Geometry: final body of the model. Coordinates: model frame, mm. Round coordinates to 2 decimals unless told otherwise and drop trailing zeros. Loops run counter-clockwise (first coordinate to the right, second up) from the corner with the lowest first, then second, coordinate; pieces in that order, holes last. Notation, with made-up numbers: (48.25, -28.5) -> (92.25, -28.5) arc R18 cw to (92.25, 1.5) -> close; hole circle Ø2 at (-38, -2.75). An arc over 180 degrees is marked (long way). Answer in a Markdown table with one row per item.
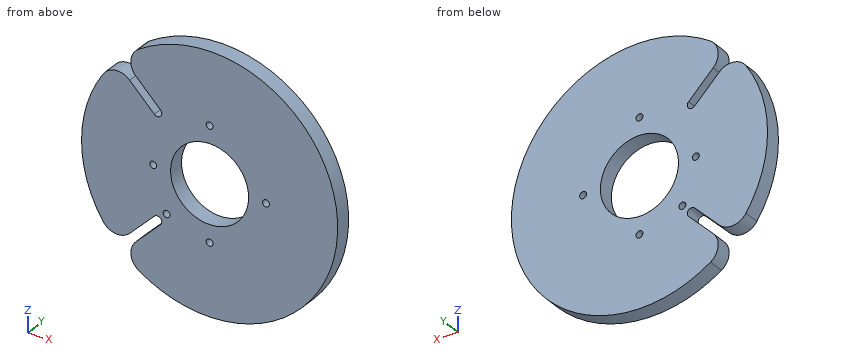
```python
from build123d import *

# Parameters (mm, degrees)
SKETCH1_R           = 75
BOSS_EXTRUDE1_DEPTH = 9.525
CUT_EXTRUDE2_REACH  = 108.493
FILLET1_R           = 10.16
SKETCH39_R          = 22.86
SKETCH39_R_2        = 2.0193
CUT_EXTRUDE30_DEPTH = 247.31360274
SKETCH42_R          = 2.0193
CUT_EXTRUDE33_DEPTH = 247.31360274


with BuildPart() as part:
    # Sketch1 → Boss-Extrude1 (new body)
    with BuildSketch(Plane(origin=(0, 0, 0), x_dir=(1, 0, 0), z_dir=(0, 1, 0))):
        with Locations(Location((0, 0, 0), (0, 0, 90))):
            Circle(SKETCH1_R)
    extrude(amount=BOSS_EXTRUDE1_DEPTH)

    # Sketch11 → Cut-Extrude2 (cut, up to next)
    with BuildSketch(Plane(origin=(0, 9.525, 0), x_dir=(1, 0, 0), z_dir=(0, 1, 0)), mode=Mode.PRIVATE) as cut_extrude2_sk1:
        with BuildLine():
            Line((-54.798637954, 51.206535505), (-32.347997651, 28.755895202))
            ThreePointArc((-32.347997651, 28.755895202), (-28.755895202, 28.755895202), (-28.755895202, 32.347997651))
            Line((-28.755895202, 32.347997651), (-51.206535505, 54.798637954))
            ThreePointArc((-51.206535505, 54.798637954), (-53.033008589, 53.033008589), (-54.798637954, 51.206535505))
        make_face()
    cut_extrude2_tool1 = extrude(cut_extrude2_sk1.sketch, amount=-CUT_EXTRUDE2_REACH, mode=Mode.PRIVATE) & part.part
    # Sketch11 → Cut-Extrude2 (cut, up to next)
    with BuildSketch(Plane(origin=(0, 9.525, 0), x_dir=(1, 0, 0), z_dir=(0, 1, 0)), mode=Mode.PRIVATE) as cut_extrude2_sk2:
        with BuildLine():
            Line((-51.206535505, -54.798637954), (-28.755895202, -32.347997651))
            ThreePointArc((-28.755895202, -32.347997651), (-28.755895202, -28.755895202), (-32.347997651, -28.755895202))
            Line((-32.347997651, -28.755895202), (-54.798637954, -51.206535505))
            ThreePointArc((-54.798637954, -51.206535505), (-53.033008589, -53.033008589), (-51.206535505, -54.798637954))
        make_face()
    cut_extrude2_tool2 = extrude(cut_extrude2_sk2.sketch, amount=-CUT_EXTRUDE2_REACH, mode=Mode.PRIVATE) & part.part
    add(cut_extrude2_tool1.solids().sort_by_distance((-41.078737, 9.525, -41.078737))[0], mode=Mode.SUBTRACT)
    add(cut_extrude2_tool2.solids().sort_by_distance((-41.078737, 9.525, 41.078737))[0], mode=Mode.SUBTRACT)

    # Fillet1
    fillet1_edges = [part.edges().sort_by_distance(p)[0] for p in [
        (-51.206535505, 4.7625, 54.798637954),
        (-54.798637954, 4.7625, 51.206535505),
        (-54.798637954, 4.7625, -51.206535505),
        (-51.206535505, 4.7625, -54.798637954),
    ]]
    fillet(fillet1_edges, radius=FILLET1_R)

    # Sketch39 → Cut-Extrude30 (cut, through all)
    with BuildSketch(Plane(origin=(-73.768816189, 9.525, -121.080352405), x_dir=(1, 0, 0), z_dir=(0, 1, 0))):
        with Locations(Location((73.768816189, -121.080352405, 0), (0, 0, 270))):
            Circle(SKETCH39_R)
        with Locations(Location((73.768816189, -88.060352405, 0), (0, 0, 270))):
            Circle(SKETCH39_R_2)
        with Locations(Location((106.788816189, -121.080352405, 0), (0, 0, 270))):
            Circle(SKETCH39_R_2)
        with Locations(Location((73.768816189, -154.100352405, 0), (0, 0, 270))):
            Circle(SKETCH39_R_2)
        with Locations(Location((40.748816189, -121.080352405, 0), (0, 0, 270))):
            Circle(SKETCH39_R_2)
    extrude(amount=-CUT_EXTRUDE30_DEPTH, mode=Mode.SUBTRACT)

    # Sketch42 → Cut-Extrude33 (cut, through all)
    with BuildSketch(Plane(origin=(-73.768816189, 9.525, -121.080352405), x_dir=(1, 0, 0), z_dir=(0, 1, 0))):
        with Locations(Location((48.605023435, -95.916559651, 0), (0, 0, 270))):
            Circle(SKETCH42_R)
    extrude(amount=-CUT_EXTRUDE33_DEPTH, mode=Mode.SUBTRACT)


solid = part.part
```
Item 1: Pin query (flat end, axial travel): pin 1 Ø1.5 at (x, y) = (-12, 7.5) entering from -Z; pin 2 Ø3 at (y, z) = (6, 43.5) entering from +X; pin 3 Ø5 at (y, z) = (1, 41.5) entering from -X; pin 4 Ø3 at (x, z) = (0, -33.02) entering from +Y. Return the tip coordinate at first contact, or that it passes through.
Answer:
| item | result |
|---|---|
| pin 1 | stops at z = -74.15 |
| pin 2 | stops at x = 62.14 |
| pin 3 | stops at x = -64.06 |
| pin 4 | passes through |
Item 2: Cut plane B-B (z = -21). Output: boundary loops of the cut face in (x, y) (3 decimals).
Answer:
| item | result |
|---|---|
| outline | (-72, 0) -> (-9.032, 0) -> (-9.032, 9.525) -> (-72, 9.525) -> close; (9.032, 0) -> (72, 0) -> (72, 9.525) -> (9.032, 9.525) -> close |
Item 3: Line query: probe 1 along X at (y, z) = (5.75, 0); probe 2 along X at (y, z) = (2.5, 33.02); probe 3 along Z at (x, y) = (-40, 8.5). Output: solid intervals per line, ascending. Write a range as [from, to].
Answer:
| item | result |
|---|---|
| probe 1 | x = [-75, -35.04], [-31, -22.86], [22.86, 31], [35.04, 75] |
| probe 2 | x = [-67.34, -36.61], [-29.43, -2.02], [2.02, 67.34] |
| probe 3 | z = [-63.44, -43.59], [-36.41, 36.41], [43.59, 63.44] |
Item 4: Cut plane A-A (x = 0). Output: boundary loops of the cut face in (y, z) (3 decimals).
Answer:
| item | result |
|---|---|
| outline | (0, -75) -> (9.525, -75) -> (9.525, -35.039) -> (0, -35.039) -> close; (0, -31.001) -> (9.525, -31.001) -> (9.525, -22.86) -> (0, -22.86) -> close; (0, 22.86) -> (9.525, 22.86) -> (9.525, 31.001) -> (0, 31.001) -> close; (0, 35.039) -> (9.525, 35.039) -> (9.525, 75) -> (0, 75) -> close |
Item 5: Cut plane D-D (y = 6). Output: boundary loops of the cut face in (x, z), then the cut area to 3 significant figures.
Answer:
| item | result |
|---|---|
| outline | (-62.39, -41.62) arc R10.16 ccw to (-46.76, -43.16) -> (-32.35, -28.76) arc R2.54 cw to (-28.76, -32.35) -> (-43.16, -46.76) arc R10.16 ccw to (-41.62, -62.39) arc R75 ccw (long way) to (-41.62, 62.39) arc R10.16 ccw to (-43.16, 46.76) -> (-28.76, 32.35) arc R2.54 cw to (-32.35, 28.76) -> (-46.76, 43.16) arc R10.16 ccw to (-62.39, 41.62) arc R75 ccw to start; hole circle Ø4.04 at (-33.02, 0); hole circle Ø4.04 at (-25.16, -25.16); hole circle Ø45.72 at (0, 0); hole circle Ø4.04 at (0, -33.02); hole circle Ø4.04 at (0, 33.02); hole circle Ø4.04 at (33.02, 0) |
| area | 15,500 mm² |
Item 6: Cut plane C-C (x = 33.02). Output: boundary loops of the cut face in (y, z) (3 decimals).
Answer:
| item | result |
|---|---|
| outline | (0, -67.34) -> (9.525, -67.34) -> (9.525, -2.019) -> (0, -2.019) -> close; (0, 2.019) -> (9.525, 2.019) -> (9.525, 67.34) -> (0, 67.34) -> close |
